```python
from build123d import *

# Parameters (mm, degrees)
SKETCH1_W               = 112
SKETCH1_H               = 200
BOSS_EXTRUDE1_DEPTH     = 5
SKETCH6_R               = 4.5
SKETCH6_R_2             = 1.95
LEANDUT_HOLES_DEPTH     = 115.721401665
CHAMFER1_SIZE           = 5
SKETCH7_R               = 50
CUT_EXTRUDE3_DEPTH      = 115.721401665
DELETEFACE1_OUTLINE_R   = 1.95
DELETEFACE1_OUTLINE_R_2 = 4.5
DELETEFACE1_DEPTH       = 5


# Read off the part's stored shape, not the designer's step: DeleteFace1
with BuildPart() as part:
    # Sketch1 → Boss-Extrude1 (new body)
    with BuildSketch(Plane.XY):
        Rectangle(SKETCH1_W, SKETCH1_H)
    extrude(amount=BOSS_EXTRUDE1_DEPTH)

    # Sketch6 → Leandut_holes (cut, through all)
    with BuildSketch(Plane.XY.offset(5)):
        with Locations((-42, 87)):
            Circle(SKETCH6_R)
        with Locations((-47.8, 92.8)):
            Circle(SKETCH6_R_2)
        with Locations(Location((-47.8, 81.2, 0), (0, 0, 180))):
            Circle(SKETCH6_R_2)
        with Locations((-36.2, 81.2)):
            Circle(SKETCH6_R_2)
        with Locations(Location((-36.2, 92.8, 0), (0, 0, 180))):
            Circle(SKETCH6_R_2)
        with Locations((36.2, 92.8)):
            Circle(SKETCH6_R_2)
        with Locations(Location((36.2, 81.2, 0), (0, 0, 180))):
            Circle(SKETCH6_R_2)
        with Locations((47.8, 81.2)):
            Circle(SKETCH6_R_2)
        with Locations(Location((47.8, 92.8, 0), (0, 0, 180))):
            Circle(SKETCH6_R_2)
        with Locations(Location((42, 87, 0), (0, 0, 180))):
            Circle(SKETCH6_R)
        with Locations((42, -87)):
            Circle(SKETCH6_R)
        with Locations((47.8, -92.8)):
            Circle(SKETCH6_R_2)
        with Locations(Location((47.8, -81.2, 0), (0, 0, 180))):
            Circle(SKETCH6_R_2)
        with Locations((36.2, -81.2)):
            Circle(SKETCH6_R_2)
        with Locations(Location((36.2, -92.8, 0), (0, 0, 180))):
            Circle(SKETCH6_R_2)
        with Locations((-36.2, -92.8)):
            Circle(SKETCH6_R_2)
        with Locations(Location((-36.2, -81.2, 0), (0, 0, 180))):
            Circle(SKETCH6_R_2)
        with Locations((-47.8, -81.2)):
            Circle(SKETCH6_R_2)
        with Locations(Location((-47.8, -92.8, 0), (0, 0, 180))):
            Circle(SKETCH6_R_2)
        with Locations(Location((-42, -87, 0), (0, 0, 180))):
            Circle(SKETCH6_R)
    extrude(amount=-LEANDUT_HOLES_DEPTH, mode=Mode.SUBTRACT)

    # Chamfer1
    chamfer1_edges = [part.edges().sort_by_distance(p)[0] for p in [
        (56, -100, 2.5),
        (-56, -100, 2.5),
        (-56, 100, 2.5),
        (56, 100, 2.5),
    ]]
    chamfer(chamfer1_edges, length=CHAMFER1_SIZE)

    # Sketch7 → Cut-Extrude3 (cut, through all)
    with BuildSketch(Plane.XY.offset(5)):
        Circle(SKETCH7_R)
    extrude(amount=-CUT_EXTRUDE3_DEPTH, mode=Mode.SUBTRACT)

    # DeleteFace1 outline → DeleteFace1 (add)
    with BuildSketch(Plane.XY):
        with Locations((-47.8, -81.2)):
            Circle(DELETEFACE1_OUTLINE_R)
        with Locations((-47.8, -92.8)):
            Circle(DELETEFACE1_OUTLINE_R)
        with Locations((-42, -87)):
            Circle(DELETEFACE1_OUTLINE_R_2)
        with Locations((36.2, 92.8)):
            Circle(DELETEFACE1_OUTLINE_R)
        with Locations((36.2, 81.2)):
            Circle(DELETEFACE1_OUTLINE_R)
        with Locations((47.8, 81.2)):
            Circle(DELETEFACE1_OUTLINE_R)
        with Locations((47.8, 92.8)):
            Circle(DELETEFACE1_OUTLINE_R)
        with Locations((-36.2, -81.2)):
            Circle(DELETEFACE1_OUTLINE_R)
        with Locations((-36.2, -92.8)):
            Circle(DELETEFACE1_OUTLINE_R)
        with Locations((42, 87)):
            Circle(DELETEFACE1_OUTLINE_R_2)
    extrude(amount=DELETEFACE1_DEPTH)


solid = part.part
```
Input: part model. Units: mm. Frame: model coordinates. Round coordinates to 2 decimals unless told otherwise and drop trailing zeros. Loops run counter-clockwise (first coordinate to the right, second up) from the corner with the lowest first, then second, coordinate; pieces in that order, holes last. Notation, with made-up numbers: (17.5, 54.5) -> (33.5, 54.5) arc R20 ccw to (33.5, 87.5) -> close; hole circle Ø2 at (79.5, 67). An arc over 180 degrees is marked (long way). One line per item, written item: value.
(1) Mould query, pull axis X, two halves, no side actions, for faces 1 (the face through (56, -1, 2)), 2 (the face through (34.4, -92.05, 2.54)), 3 (the face through (-56, -1, 2)), 4 (the face through (-51, 1, 5)). Classes: pulls with the +X half, pulls with the -X half, needs draft (parallel to the pull), parting line crosses it, or undercut.
Geometry check:
face 1: pulls with the +X half
face 2: undercut
face 3: pulls with the -X half
face 4: needs draft
(2) Section A-A (x = 0). Return the cut outline in (y, z), plus the area to 3 significant figures.
Geometry check:
outline: (-100, 0) -> (-50, 0) -> (-50, 5) -> (-100, 5) -> close; (50, 0) -> (100, 0) -> (100, 5) -> (50, 5) -> close
area: 500 mm2
(3) Material intervals for line 1 (Y direction, x = 42, z = 3.75); line 2 (Y direction, x = -36.2, z = 3.6); line 3 (Y direction, x = 0, z = 2.75), sorted ascending. Write a range as [from, to].
Geometry check:
line 1: [-100, -91.5], [-82.5, -27.13], [27.13, 100]
line 2: [-100, -34.49], [34.49, 79.25], [83.15, 90.85], [94.75, 100]
line 3: [-100, -50], [50, 100]
(4) Section D-D (x = 42). Return the cut outline in (y, z).
Geometry check:
outline: (-100, 0) -> (-91.5, 0) -> (-91.5, 5) -> (-100, 5) -> close; (-82.5, 0) -> (-27.13, 0) -> (-27.13, 5) -> (-82.5, 5) -> close; (27.13, 0) -> (100, 0) -> (100, 5) -> (27.13, 5) -> close
(5) Section B-B (y = -87). Return the cut outline in (x, z), plus the area to 3 significant figures.
Geometry check:
outline: (-56, 0) -> (37.5, 0) -> (37.5, 5) -> (-56, 5) -> close; (46.5, 0) -> (56, 0) -> (56, 5) -> (46.5, 5) -> close
area: 515 mm2
(6) Section C-C (z = 1.1). Give the number of separate pieces and of enclosed holes in the cut face, plus the area to 3 significant figures.
Geometry check:
separate pieces: 1
enclosed holes: 11
area: 14,300 mm2
(7) Pin query (flat end, axial travel): pin 1 (2.5 mm diameter, centred on x = 47.8, y = -92.8, fed in from -Z). Return the tip coordinate at first contact, or that it passes through.
Geometry check:
pin 1: through
